Geometry: final body of the model. Coordinates: model frame, mm. Face numbers are marked on the shaded views. Coordinates: 2 decimals unless noted, no trailing zeros. Order: outer loops, then holes, each group sorted by start corner. A loop starts at its lowest first (then second) coordinate and runs counter-clockwise, first axis right, second up. Notation, with made-up numbers: M -8.75,-26.5 L 16.25,-26.5 A20 cw 16.25,4.5 Z; hole C 28,7.25 d8. An arc over 180 degrees is marked long. One line per question, with ' | ' between items.
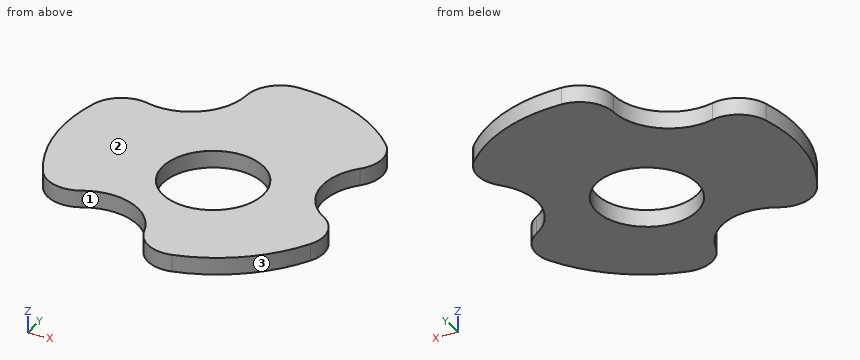
from build123d import *

# Parameters (mm, degrees)
F0_R     = 56.7715385185
F1_DEPTH = 6.35
F2_R     = 18.6477696788
F3_DEPTH = 25.4
F5_DEPTH = 25.4
F6_R     = 12.7


with BuildPart() as f1:
    # F0 (on Top) → F1 (new body)
    with BuildSketch(Plane.XY):
        Circle(F0_R)
    extrude(amount=F1_DEPTH)

    # F2 (on face) → F3 (cut)
    with BuildSketch(Plane.XY.offset(6.35)):
        with Locations((2.8365715407, -7.6775541529)):
            Circle(F2_R)
    extrude(amount=-F3_DEPTH, mode=Mode.SUBTRACT)

    # F4 (on face) → F5 (cut)
    with BuildSketch(Plane.XY.offset(6.35)):
        with BuildLine():
            ThreePointArc((-16.6661772977, 54.2701217987), (-35.2620612858, 44.4926355663), (-49.0286391406, 28.6216723792))
            ThreePointArc((-49.0286391406, 28.6216723792), (-22.2124908393, 28.0270699981), (-16.6661772977, 54.2701217987))
        make_face()
        with BuildLine():
            ThreePointArc((56.7715385185, 0), (54.8722368944, 14.5617720065), (49.3014149495, 28.1492108191))
            ThreePointArc((49.3014149495, 28.1492108191), (35.3784000316, 5.2230463491), (55.332392793, -12.7017279755))
            ThreePointArc((55.332392793, -12.7017279755), (56.4106047412, -6.391498924), (56.7715385185, 0))
        make_face()
        with BuildLine():
            ThreePointArc((-0.2727758089, -56.7708831983), (-13.1659091923, -33.2501163472), (-38.6662154953, -41.5683938231))
            ThreePointArc((-38.6662154953, -41.5683938231), (-20.9007220389, -52.7841586465), (-0.2727758089, -56.7708831983))
        make_face()
    extrude(amount=-F5_DEPTH, mode=Mode.SUBTRACT)

    # F6
    f6_edges = [f1.edges().sort_by_distance(p)[0] for p in [
        (-0.272776, -56.770883, 3.175),
        (-38.666215, -41.568394, 3.175),
        (49.301415, 28.149211, 3.175),
        (55.332393, -12.701728, 3.175),
        (-16.666177, 54.270122, 3.175),
        (-49.028639, 28.621672, 3.175),
    ]]
    fillet(f6_edges, radius=F6_R)


solid = f1.part
1. Draft query along X for the marked faces 1, 2 and 3. Return one class per face: pulls with the +X half, pulls with the -X half, needs draft (parallel to the pull), parting line crosses it, or undercut.
Response values:
face 1: undercut | face 2: needs draft | face 3: pulls with the +X half
2. Material intervals for line 1 (X direction, y = -18, z = 5.25); line 2 (X direction, y = -15, z = 5.5); line 3 (Y direction, x = 0, z = 4.75), sorted ascending. Write a range as [from, to].
Response values:
line 1: x = [-53.84, -12.69], [18.37, 51.34] | line 2: x = [-54.75, -14.31], [19.99, 50.28] | line 3: y = [-48.53, -26.11], [10.75, 56.77]
3. Section B-B, the plane x = -20.5. Output: boundary loops of the cut face in (y, z), and give its area (3 significant figures).
Response values:
outline: M -31.78,0 L 29.54,0 L 29.54,6.35 L -31.78,6.35 Z | area: 389 mm^2
4. Section A-A, the plane x = 36.5. Output: boundary loops of the cut face in (y, z).
Response values:
outline: M -43.48,0 L 0.89,0 L 0.89,6.35 L -43.48,6.35 Z; M 15.69,0 L 43.48,0 L 43.48,6.35 L 15.69,6.35 Z
